Verification items for the finished model (mm, model axes). A direction names the side the tool comes from. Give positions to 0.01 mm unless a question says otherwise; leave off trailing zeros. Write each loop counter-clockwise with the first axis right and the second up, starting at its lowest first coordinate (ties: lowest second). Pieces come first, ordered by that corner, then holes. Notation, with made-up numbers: (57, -14) -> (116, -14) arc R20 ccw to (116, 0) -> close; hole circle Ø7 at (58.25, 28). An arc over 180 degrees is marked (long way). Use one line per item in the form item = value. Start each with the question number.
(1) Section check A-A, the plane x = 0. Record the cut outline in (y, z).
(2) Release check for a two-part mould opening along X. For faces 1 (the face through (2, 0, 0)), 2 (the face through (0, -1, 1)), 3 (the face through (-5.5, 5.1, 4.9)) record: pulls with the +X half, pulls with the -X half, needs draft (parallel to the pull), parting line crosses it, or undercut.
(3) Section check B-B, the plane z = 4. Record the cut outline in (x, y).
(4) Set-up check for faces 4 (the face through (-0.1, -4.3, 5)), 5 (the face through (-6, -3, 5)), 6 (the face through (0, -7, 1.5)): record each of +Z, -Z, +X, -X, +Y, -Y from which the full face is reachable in a straight line by a thin tool's end or side.
(5) Section check C-C, the plane y = 0.5. Record the cut outline in (x, z), plus the area to 3 significant figures.
(6) Scan lines: L1, parallel to Z at x = -1, y = 3.5; L2, parallel to Y at x = 0, z = 9.15; L3, parallel to Z at x = -5.5, y = -4. Record each from-to range of solid material in increasing order.
(7) Depth check by flat-ended pin: pin 1 Ø1.5 at (y, z) = (1.5, 5.5) entering from -X; pin 2 Ø1.2 at (x, z) = (6.5, 4) entering from -Y; pin 3 Ø1.5 at (x, z) = (-3, 8) entering from -Y. Enter the tip coordinate at first touch or a pass-through.
(8) Section check D-D, the plane z = 8.75. Record the cut outline in (x, y), plus the area to 3 significant figures.
from build123d import *

# Parameters (mm, degrees)
SKETCH_1_R          = 7.5
EXTRUDE_1_DEPTH     = 10
CUT_EXTRUDE_1_DEPTH = 5
SKETCH_3_R          = 1
CUT_EXTRUDE_2_DEPTH = 15.577379737
CUT_EXTRUDE_3_DEPTH = 7


with BuildPart() as part:
    # 草图1 → 凸台-拉伸1 (new body)
    with BuildSketch(Plane.XY):
        Circle(SKETCH_1_R)
    extrude(amount=EXTRUDE_1_DEPTH)

    # 草图2 → 切除-拉伸1 (cut)
    with BuildSketch(Plane(origin=(0, 0, 2.5), x_dir=(-1, 0, 0), z_dir=(0, 0, -1))):
        with BuildLine():
            Line((-4.3, 0), (-4.3, 6.144916598))
            ThreePointArc((-4.3, 6.144916598), (0, 7.5), (4.3, 6.144916598))
            Line((4.3, 6.144916598), (4.3, 0))
            ThreePointArc((4.3, 0), (0, -4.3), (-4.3, 0))
        make_face()
    extrude(amount=-CUT_EXTRUDE_1_DEPTH, mode=Mode.SUBTRACT)

    # 草图3 → 切除-拉伸2 (cut, through all)
    with BuildSketch(Plane(origin=(0, 0, 0), x_dir=(-1, 0, 0), z_dir=(0, 0, -1))):
        Circle(SKETCH_3_R)
    extrude(amount=-CUT_EXTRUDE_2_DEPTH, mode=Mode.SUBTRACT)

    # 草图5 → 切除-拉伸3 (cut)
    with BuildSketch(Plane(origin=(0, 0, 1.5), x_dir=(-1, 0, 0), z_dir=(0, 0, -1))):
        with BuildLine():
            Line((-5.766281297, -3), (-6.873863542, -3))
            ThreePointArc((-6.873863542, -3), (0, -7.5), (6.873863542, -3))
            Line((6.873863542, -3), (5.766281297, -3))
            ThreePointArc((5.766281297, -3), (0, -6.5), (-5.766281297, -3))
        make_face()
    extrude(amount=-CUT_EXTRUDE_3_DEPTH, mode=Mode.SUBTRACT)


solid = part.part
Completed:
q1.outline = (-7.5, 0) -> (-1, 0) -> (-1, 2.5) -> (-4.3, 2.5) -> (-4.3, 7.5) -> (-1, 7.5) -> (-1, 10) -> (-7.5, 10) -> (-7.5, 8.5) -> (-6.5, 8.5) -> (-6.5, 1.5) -> (-7.5, 1.5) -> close; (1, 0) -> (7.5, 0) -> (7.5, 2.5) -> (1, 2.5) -> close; (1, 7.5) -> (7.5, 7.5) -> (7.5, 10) -> (1, 10) -> close
q2.face_1 = needs draft
q2.face_2 = undercut
q2.face_3 = parting line crosses it
q3.outline = (-6.87, -3) -> (-5.77, -3) arc R6.5 ccw to (5.77, -3) -> (6.87, -3) arc R7.5 ccw to (4.3, 6.14) -> (4.3, 0) arc R4.3 cw to (-4.3, 0) -> (-4.3, 6.14) arc R7.5 ccw to start
q4.face_4 = +Y
q4.face_5 = -X, -Y
q4.face_6 = -Y
q5.outline = (-7.48, 0) -> (-0.87, 0) -> (-0.87, 2.5) -> (-4.3, 2.5) -> (-4.3, 7.5) -> (-0.87, 7.5) -> (-0.87, 10) -> (-7.48, 10) -> close; (0.87, 0) -> (7.48, 0) -> (7.48, 10) -> (0.87, 10) -> (0.87, 7.5) -> (4.3, 7.5) -> (4.3, 2.5) -> (0.87, 2.5) -> close
q5.area = 98.0 mm²
q6.L1 = 0 to 2.5, 7.5 to 10
q6.L2 = -7.5 to -1, 1 to 7.5
q6.L3 = 0 to 1.5, 8.5 to 10
q7.pin_1 = -7.46
q7.pin_2 = -3
q7.pin_3 = -7.09
q8.outline = circle Ø15 at (0, 0); hole circle Ø2 at (0, 0)
q8.area = 174 mm²
